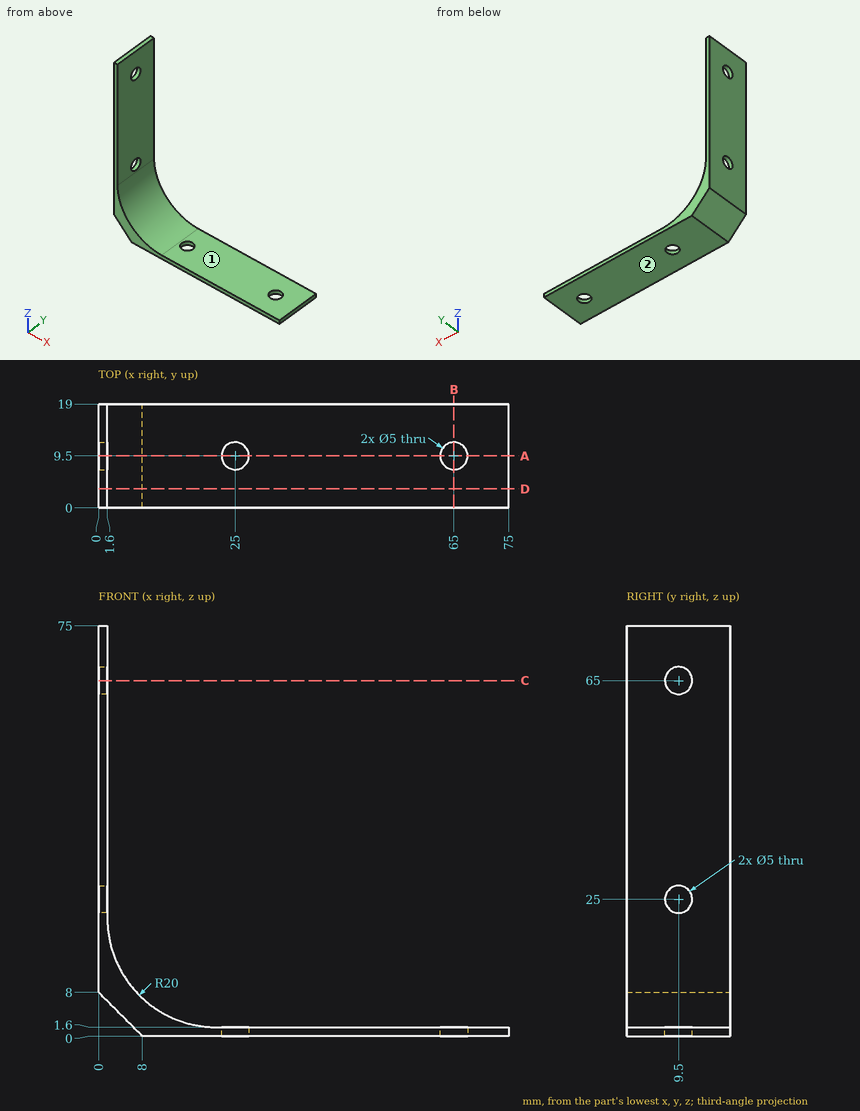
Design review of the part shown in the three views and the two pictorial views. Dimensions are in mm from the part's minimum x, y and z. A direction names the side the tool comes from. Round coordinates to 2 decimals unless told otherwise and drop trailing zeros. Loops run counter-clockwise (first coordinate to the right, second up) from the corner with the lowest first, then second, coordinate; pieces in that order, holes last. Notation, with made-up numbers: M 52.5,-1.5 L 95.5,-1.5 A34 ccw 95.5,35.5 Z; hole C 89,7.25 d10. An arc over 180 degrees is marked long. Answer as a JSON object with one key per item and string values.
Item 1: Clearance check with flat-ended pins moving along their axes: P1, Ø5.5, axis at y = 12.5, z = 57, coming from the +X side; P2, Ø2, axis at x = 30, y = 9, coming from the +Z side. State where each tip first meets the part, or that it passes through.
Check sheet entries:
{"P1": "x = 1.6", "P2": "z = 1.6"}
Item 2: We need section C-C, the plane z = 65. State the section outline as (x, y) points.
Check sheet entries:
{"outline": "M 0,0 L 1.6,0 L 1.6,7 L 0,7 Z; M 0,12 L 1.6,12 L 1.6,19 L 0,19 Z"}
Item 3: For line 1 along Y through (x, z) = (25, 0.65); line 2 along X through (y, z) = (8.25, 34.5), list the stretches that pass through material, from the lowest coordinate up.
Check sheet entries:
{"line 1": "0 to 7, 12 to 19", "line 2": "0 to 1.6"}
Item 4: We need section D-D, the plane y = 3.5. State the section outline as (x, z) points, and give its area (3 significant figures).
Check sheet entries:
{"outline": "M 0,8 L 8,0 L 75,0 L 75,1.6 L 21.6,1.6 A20 cw 1.6,21.6 L 1.6,75 L 0,75 Z", "area": "291 mm2"}
Item 5: We need section A-A, the plane y = 9.5. State the section outline as (x, z) points.
Check sheet entries:
{"outline": "M 0,8 L 8,0 L 22.5,0 L 22.5,1.6 L 21.6,1.6 A20 cw 1.6,21.6 L 1.6,22.5 L 0,22.5 Z; M 0,27.5 L 1.6,27.5 L 1.6,62.5 L 0,62.5 Z; M 0,67.5 L 1.6,67.5 L 1.6,75 L 0,75 Z; M 27.5,0 L 62.5,0 L 62.5,1.6 L 27.5,1.6 Z; M 67.5,0 L 75,0 L 75,1.6 L 67.5,1.6 Z"}
Item 6: Tool access review of the marked faces 1 and 2: name each direction out of +Z, -Z, +X, -X, +Y, -Y from which nothing blocks a thin tool from reaching the whole face with its end or side.
Check sheet entries:
{"face 1": "+Z, +X, +Y, -Y", "face 2": "-Z, +X, -X, +Y, -Y"}
Item 7: We need section B-B, the plane x = 65. State the section outline as (y, z) points.
Check sheet entries:
{"outline": "M 0,0 L 7,0 L 7,1.6 L 0,1.6 Z; M 12,0 L 19,0 L 19,1.6 L 12,1.6 Z"}
